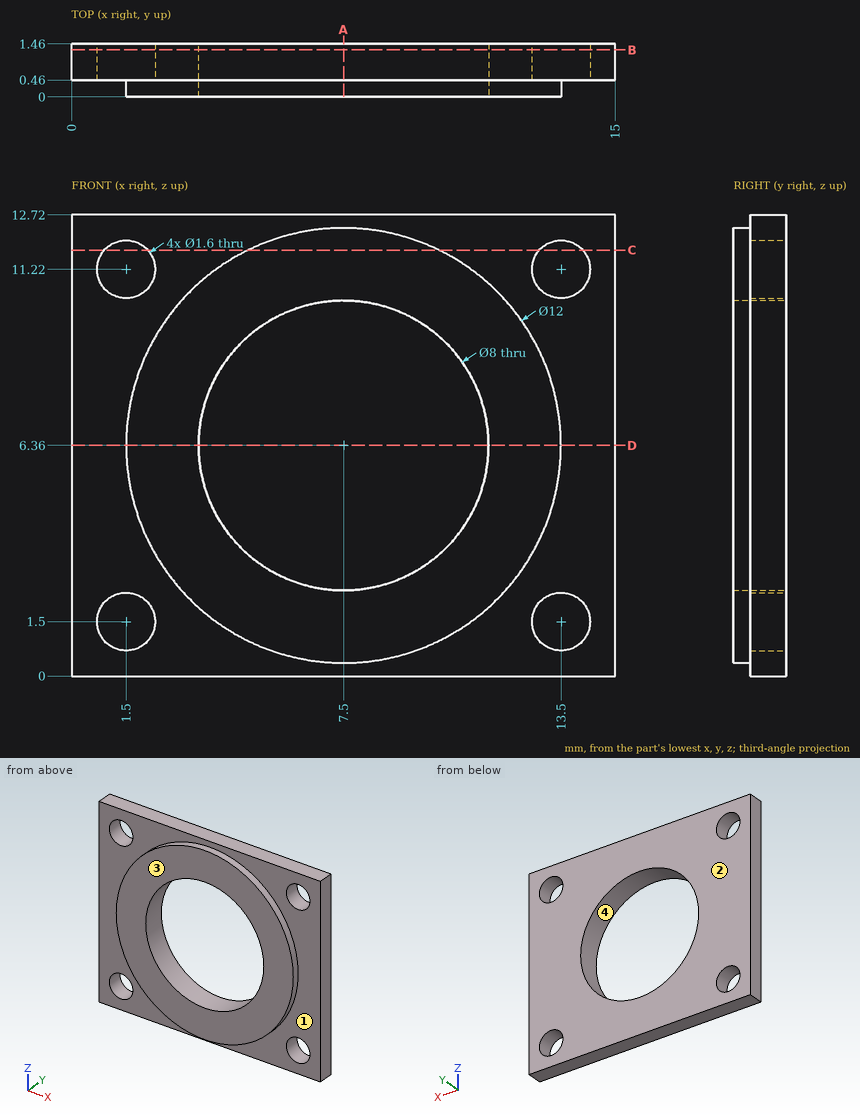
Drawing for the job (mm, zero at the part's lowest x, y, z). A direction names the side the tool comes from. Round coordinates to 2 decimals unless told otherwise and drop trailing zeros. Loops run counter-clockwise (first coordinate to the right, second up) from the corner with the lowest first, then second, coordinate; pieces in that order, holes last.
1. Wall check: probe 1 along Z at (x, y) = (13.5, 0.7); probe 2 along X at (y, z) = (0.7, 11.22); probe 3 along X at (y, z) = (0.8, 6.5). Give the ranges that are in metal, low to high.
Check values:
probe 1: z = 0 to 0.7, 2.3 to 10.42, 12.02 to 12.72
probe 2: x = 0 to 0.7, 2.3 to 12.7, 14.3 to 15
probe 3: x = 0 to 3.5, 11.5 to 15
2. Drop a flat-ended pin along its axis: P1, Ø1, axis at x = 1.5, z = 1.5, coming from the -Y side (3 decimals). Give the stop position or say it passes through.
Check values:
P1: passes through
3. Band-saw the part on C-C, the plane z = 11.75. List the corners of the cut face in (x, y).
Check values:
outline: (0, 0.46) - (0.9, 0.46) - (0.9, 1.46) - (0, 1.46) - close; (2.1, 0.46) - (4.86, 0.46) - (4.86, 0) - (10.14, 0) - (10.14, 0.46) - (12.9, 0.46) - (12.9, 1.46) - (2.1, 1.46) - close; (14.1, 0.46) - (15, 0.46) - (15, 1.46) - (14.1, 1.46) - close
4. Mould opens along Z. For the marked faces 3 and 4 say: +Z half, -Z half, draft (parallel to the pull), parting line (faces both ways), or undercut.
Check values:
face 3: draft
face 4: undercut
5. Tool access for the marked faces 1 and 2: list every direction of +Z, -Z, +X, -X, +Y, -Y with a clear straight run to the whole face (end or side of a thin tool).
Check values:
face 1: -Y
face 2: +Z, -Z, +X, -X, +Y
6. Band-saw the part on B-B, the plane y = 1.3. List the corners of the cut face in (x, z).
Check values:
outline: (0, 0) - (15, 0) - (15, 12.72) - (0, 12.72) - close; hole circle Ø1.6 at (1.5, 1.5); hole circle Ø1.6 at (1.5, 11.22); hole circle Ø8 at (7.5, 6.36); hole circle Ø1.6 at (13.5, 1.5); hole circle Ø1.6 at (13.5, 11.22)
7. Band-saw the part on A-A, the plane x = 7.5. List the corners of the cut face in (y, z).
Check values:
outline: (0, 0.36) - (0.46, 0.36) - (0.46, 0) - (1.46, 0) - (1.46, 2.36) - (0, 2.36) - close; (0, 10.36) - (1.46, 10.36) - (1.46, 12.72) - (0.46, 12.72) - (0.46, 12.36) - (0, 12.36) - close
8. Band-saw the part on D-D, the plane z = 6.36. List the corners of the cut face in (x, y).
Check values:
outline: (0, 0.46) - (1.5, 0.46) - (1.5, 0) - (3.5, 0) - (3.5, 1.46) - (0, 1.46) - close; (11.5, 0) - (13.5, 0) - (13.5, 0.46) - (15, 0.46) - (15, 1.46) - (11.5, 1.46) - close
